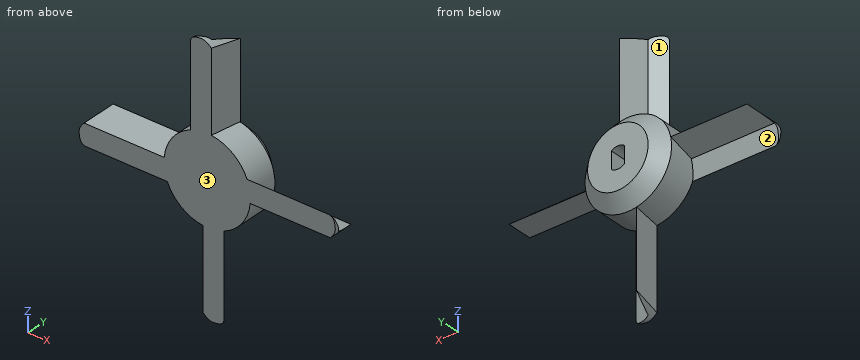
```python
from build123d import *

# Parameters (mm, degrees)
SKETCH1_R           = 10
BOSS_EXTRUDE2_DEPTH = 10
CIRPATTERN1_COUNT   = 4
CUT_EXTRUDE3_DEPTH  = 6.15
CUT_EXTRUDE4_DEPTH  = 8.45
CIRPATTERN2_COUNT   = 4
CHAMFER1_SIZE       = 3


with BuildPart() as part:
    # Sketch1 → Boss-Extrude2 (new body)
    with BuildSketch(Plane(origin=(0, 0, 0), x_dir=(1, 0, 0), z_dir=(0, 1, 0))):
        with Locations(Location((0, 0, 0), (0, 0, 270))):
            Circle(SKETCH1_R)
    extrude(amount=BOSS_EXTRUDE2_DEPTH)

    # Sketch2 → Loft1 section 0
    with BuildSketch(Plane.XY.offset(8)):
        with BuildLine():
            Line((0, 1.334072036), (1.933158154, 7.086396301))
            Line((1.933158154, 7.086396301), (0.966579077, 0))
            Line((0.966579077, 0), (-3.866316309, 0))
            Line((-3.866316309, 0), (0, 1.334072036))
        make_face()
    # Sketch3 → Loft1 section 1
    with BuildSketch(Plane.XY.offset(30)):
        with BuildLine():
            Line((0, 1.334072036), (1.933158154, 7.086396301))
            Line((1.933158154, 7.086396301), (0.966579077, 0))
            Line((0.966579077, 0), (-3.866316309, 0))
            Line((-3.866316309, 0), (0, 1.334072036))
        make_face()
    loft1 = loft()

    # CirPattern1: Loft1 ×4 about axis
    cirpattern1_axis = Axis((0, 0, 0), (0, 1, 0))
    for i in range(1, CIRPATTERN1_COUNT):
        add(loft1.rotate(cirpattern1_axis, i * 360 / CIRPATTERN1_COUNT))

    # Sketch8 → Cut-Extrude3 (cut)
    with BuildSketch(Plane(origin=(0, 10, 0), x_dir=(1, 0, 0), z_dir=(0, 1, 0))):
        with BuildLine():
            Line((1.5, 1.968660712), (1.5, -1.968660712))
            ThreePointArc((1.5, -1.968660712), (0, -2.475), (-1.5, -1.968660712))
            Line((-1.5, -1.968660712), (-1.5, 1.968660712))
            ThreePointArc((-1.5, 1.968660712), (0, 2.475), (1.5, 1.968660712))
        make_face()
    extrude(amount=-CUT_EXTRUDE3_DEPTH, mode=Mode.SUBTRACT)

    # Sketch9 → Cut-Extrude4 (cut)
    with BuildSketch(Plane.XZ):
        with BuildLine():
            Line((28.274704093, 3.866316309), (30.023429762, 3.866316309))
            Line((30.023429762, 3.866316309), (30.023429762, -1.933158154))
            Line((30.023429762, -1.933158154), (27.489632408, -1.933158154))
            add(Edge.make_bspline(
                [(28.274704093, 3.866316309), (29.251563836, 3.579912726), (29.503721472, 2.469841159), (29.781293332, 0.089495711), (28.257519324, -1.153109295), (27.489632408, -1.933158154)],
                knots=[0, 0, 0, 0, 0.329035363, 0.48426931, 1, 1, 1, 1], degree=3))
        make_face()
    cut_extrude4 = extrude(amount=-CUT_EXTRUDE4_DEPTH, mode=Mode.SUBTRACT)

    # CirPattern2: Cut-Extrude4 ×4 about axis
    cirpattern2_axis = Axis((0, 10, 0), (0, 1, 0))
    for i in range(1, CIRPATTERN2_COUNT):
        add(cut_extrude4.rotate(cirpattern2_axis, i * 360 / CIRPATTERN2_COUNT), mode=Mode.SUBTRACT)

    # Chamfer1
    # the kernel refuses this chamfer: 3 mm, written as the material it takes off along each edge
    with BuildSketch(Plane(origin=(0, 10, 0), x_dir=(0, 0, 1), z_dir=(-1, 0, 0))) as chamfer1_piece_1_section:
        Polygon((10, -CHAMFER1_SIZE), (10 - CHAMFER1_SIZE, 0), (10, 0), align=None)
    chamfer1_piece_1 = revolve(axis=Axis((0, 10, 0), (0, 1, 0)), mode=Mode.PRIVATE)
    chamfer1_piece_1 = split(chamfer1_piece_1, bisect_by=Plane(origin=(2.324578556, 8.251110666, 8.890331171), z_dir=(-0.947903464475993, 0.3185577216681616, 0)), keep=Keep.TOP, mode=Mode.PRIVATE)
    chamfer1_piece_1 = split(chamfer1_piece_1, bisect_by=Plane(origin=(-2.324578556, 8.251110666, 8.890331171), z_dir=(0.947903464475993, 0.3185577216681616, 0)), keep=Keep.TOP, mode=Mode.PRIVATE)
    add(chamfer1_piece_1, mode=Mode.SUBTRACT)
    with BuildSketch(Plane(origin=(0, 10, 0), x_dir=(0, 0, 1), z_dir=(-1, 0, 0))) as chamfer1_piece_2_section:
        Polygon((10, -CHAMFER1_SIZE), (10 - CHAMFER1_SIZE, 0), (10, 0), align=None)
    chamfer1_piece_2 = revolve(axis=Axis((0, 10, 0), (0, 1, 0)), mode=Mode.PRIVATE)
    chamfer1_piece_2 = split(chamfer1_piece_2, bisect_by=Plane(origin=(-1.927187537, 7.042623199, 9.791355143), z_dir=(0.9908254446191594, 0.13514783866287053, 0)), keep=Keep.TOP, mode=Mode.PRIVATE)
    chamfer1_piece_2 = split(chamfer1_piece_2, bisect_by=Plane(origin=(-1.922954088, 3.507226982, -0.730322564), z_dir=(0, 0.3185577216681616, 0.947903464475993)), keep=Keep.TOP, mode=Mode.PRIVATE)
    chamfer1_piece_2 = split(chamfer1_piece_2, bisect_by=Plane(origin=(-1.919079209, 7.044502852, 9.791355143), z_dir=(-0.947903464475993, -0.3185577216681616, 0)), keep=Keep.TOP, mode=Mode.PRIVATE)
    add(chamfer1_piece_2, mode=Mode.SUBTRACT)
    with BuildSketch(Plane(origin=(0, 10, 0), x_dir=(0, 0, 1), z_dir=(-1, 0, 0))) as chamfer1_piece_3_section:
        Polygon((10, -CHAMFER1_SIZE), (10 - CHAMFER1_SIZE, 0), (10, 0), align=None)
    chamfer1_piece_3 = revolve(axis=Axis((0, 10, 0), (0, 1, 0)), mode=Mode.PRIVATE)
    chamfer1_piece_3 = split(chamfer1_piece_3, bisect_by=Plane(origin=(2.255597721, 9.450335897, 6.172482093), z_dir=(0.9908254446191594, -0.13514783866287053, 0)), keep=Keep.TOP, mode=Mode.PRIVATE)
    chamfer1_piece_3 = split(chamfer1_piece_3, bisect_by=Plane(origin=(6.172482093, 6.28280667, -1.663099344), z_dir=(0, 0.3185577216681616, 0.947903464475993)), keep=Keep.TOP, mode=Mode.PRIVATE)
    add(chamfer1_piece_3, mode=Mode.SUBTRACT)
    with BuildSketch(Plane(origin=(0, 10, 0), x_dir=(0, 0, 1), z_dir=(-1, 0, 0))) as chamfer1_piece_4_section:
        Polygon((10, -CHAMFER1_SIZE), (10 - CHAMFER1_SIZE, 0), (10, 0), align=None)
    chamfer1_piece_4 = revolve(axis=Axis((0, 10, 0), (0, 1, 0)), mode=Mode.PRIVATE)
    chamfer1_piece_4 = split(chamfer1_piece_4, bisect_by=Plane(origin=(-6.172482093, 9.450335897, 2.255597721), z_dir=(0, -0.13514783866287053, 0.9908254446191594)), keep=Keep.TOP, mode=Mode.PRIVATE)
    chamfer1_piece_4 = split(chamfer1_piece_4, bisect_by=Plane(origin=(-2.915854237, 10.010516351, 6.172482093), z_dir=(-0.947903464475993, -0.3185577216681616, 0)), keep=Keep.TOP, mode=Mode.PRIVATE)
    add(chamfer1_piece_4, mode=Mode.SUBTRACT)
    with BuildSketch(Plane(origin=(0, 10, 0), x_dir=(0, 0, 1), z_dir=(-1, 0, 0))) as chamfer1_piece_5_section:
        Polygon((10, -CHAMFER1_SIZE), (10 - CHAMFER1_SIZE, 0), (10, 0), align=None)
    chamfer1_piece_5 = revolve(axis=Axis((0, 10, 0), (0, 1, 0)), mode=Mode.PRIVATE)
    chamfer1_piece_5 = split(chamfer1_piece_5, bisect_by=Plane(origin=(-2.32080528, 9.928399838, 0), z_dir=(-0.9908254446191594, -0.13514783866287053, 0)), keep=Keep.TOP, mode=Mode.PRIVATE)
    chamfer1_piece_5 = split(chamfer1_piece_5, bisect_by=Plane(origin=(-8.890331171, 8.251110666, 2.324578556), z_dir=(0, 0.3185577216681616, -0.947903464475993)), keep=Keep.TOP, mode=Mode.PRIVATE)
    add(chamfer1_piece_5, mode=Mode.SUBTRACT)
    with BuildSketch(Plane(origin=(0, 10, 0), x_dir=(0, 0, 1), z_dir=(-1, 0, 0))) as chamfer1_piece_6_section:
        Polygon((10, -CHAMFER1_SIZE), (10 - CHAMFER1_SIZE, 0), (10, 0), align=None)
    chamfer1_piece_6 = revolve(axis=Axis((0, 10, 0), (0, 1, 0)), mode=Mode.PRIVATE)
    chamfer1_piece_6 = split(chamfer1_piece_6, bisect_by=Plane(origin=(6.172482093, 9.450335897, -2.255597721), z_dir=(0, -0.13514783866287053, -0.9908254446191594)), keep=Keep.TOP, mode=Mode.PRIVATE)
    chamfer1_piece_6 = split(chamfer1_piece_6, bisect_by=Plane(origin=(-1.663099344, 6.28280667, -6.172482093), z_dir=(0.947903464475993, 0.3185577216681616, 0)), keep=Keep.TOP, mode=Mode.PRIVATE)
    add(chamfer1_piece_6, mode=Mode.SUBTRACT)


solid = part.part
```
Geometry check sheet. Reference: the model listing, model coordinates, mm. Face numbers are marked on the shaded views. A direction names the side the tool comes from. Give positions to 0.01 mm unless a question says otherwise; leave off trailing zeros. Order: outer loops, then holes, each group sorted by start corner. A loop starts at its lowest first (then second) coordinate and runs counter-clockwise, first axis right, second up. Notation, with made-up numbers: (62, 41.5) - (71, 41.5) arc R16 ccw to (71, 57.5) - close; hole circle Ø5 at (-31, 3). An arc over 180 degrees is marked (long way). Answer in a Markdown table with one row per item. Add a question column.
Q1. Gauge pin test, flat ends, axial feed: pin 1 (1.5 mm diameter, centred on x = -1, y = 7, fed in from -Z); pin 2 (6 mm diameter, centred on y = 2, z = -22.5, fed in from -X); pin 3 (2 mm diameter, centred on y = 7, z = -1, fed in from +X). Record the tip position at first contact, or that the pin passes through.
Q2. Material ranges on probe 1 along Z at (x, y) = (2, 1.25); probe 2 along Z at (x, y) = (-7.5, 3.75); probe 3 along X at (y, z) = (6.5, -5), recorded low to high. Write a range as from..to.
Q3. Cross-section at A-A, the plane x = 20. Enter the section's corners in (y, z).
Q4. Tool access check on the marked faces 1, 2 and 3. Record the directions out of +Z, -Z, +X, -X, +Y, -Y that give a thin tool (end or side, any length) a straight path to the whole face; none if there is none.
Q5. Cross-section at B-B, the plane z = -17.5. Enter the section's corners in (x, y), then the cut area to 3 significant figures.
Check values:
| question | item | result |
|---|---|---|
| 1 | pin 1 | stops at z = -10 |
| 1 | pin 2 | stops at x = -1.65 |
| 1 | pin 3 | stops at x = 27.78 |
| 2 | probe 1 | z = -9.8..9.8 |
| 2 | probe 2 | z = -6.61..6.61 |
| 2 | probe 3 | x = -8.66..8.66 |
| 3 | outline | (0, -0.97) - (7.09, -1.93) - (1.33, 0) - (0, 3.87) - close |
| 4 | face 1 | +Z, -X, +Y |
| 4 | face 2 | -Z, -X, +Y |
| 4 | face 3 | +Z, -Z, +X, -X, -Y |
| 5 | outline | (-1.93, 7.09) - (-0.97, 0) - (3.87, 0) - (0, 1.33) - close |
| 5 | area | 7.29 mm^2 |
